Autodesk Inventor part; units mm, degrees
ref_plane "YZ Plane" through (0, 0, 0) normal (1, 0, 0) x (0, 1, 0)
ref_plane "XZ Plane" through (0, 0, 0) normal (0, 1, 0) x (-1, 0, 0)
ref_plane "XY Plane" through (0, 0, 0) normal (0, 0, 1) x (1, 0, 0)
sketch "Sketch1" plane through (0, 0, 0) normal (0, 1, 0) x (-1, 0, 0)
  point P0 (0, 0)
sketch "Sketch2" plane through (0, 0, 0) normal (0, 1, 0) x (-1, 0, 0)
  circle A0 centre (0, 0) radius 6.35 construction
  circle A1 centre (0, -44.45) radius 38.1 construction
  circle A2 centre (0, 0) radius 25.4 construction
  circle A3 centre (17.9605, -17.9605) radius 2.4892 construction
  circle A4 centre (25.4, 0) radius 2.4892 construction
  circle A5 centre (17.9605, 17.9605) radius 2.4892 construction
  circle A6 centre (0, 25.4) radius 2.4892 construction
  circle A7 centre (-17.9605, 17.9605) radius 2.4892 construction
  circle A8 centre (-25.4, 0) radius 2.4892 construction
  circle A9 centre (-17.9605, -17.9605) radius 2.4892 construction
  circle A10 centre (0, -25.4) radius 2.4892 construction
  circle A11 centre (0, -88.9) radius 25.4 construction
  circle A12 centre (0, -88.9) radius 6.35 construction
  circle A13 centre (-17.9605, -70.9395) radius 2.4892 construction
  circle A14 centre (-25.4, -88.9) radius 2.4892 construction
  circle A15 centre (-17.9605, -106.8605) radius 2.4892 construction
  circle A16 centre (0, -114.3) radius 2.4892 construction
  circle A17 centre (17.9605, -106.8605) radius 2.4892 construction
  circle A18 centre (25.4, -88.9) radius 2.4892 construction
  circle A19 centre (17.9605, -70.9395) radius 2.4892 construction
  circle A20 centre (0, -63.5) radius 2.4892 construction
  circle A21 centre (0, 0) radius 9.525 construction
  circle A22 centre (0, -88.9) radius 9.525 construction
  circle A23 centre (47.3968, -12.5178) radius 6.35 construction
  circle A24 centre (47.3968, -76.3822) radius 6.35 construction
  circle A25 centre (-47.3968, -76.3822) radius 6.35 construction
  circle A26 centre (0, 0) radius 29.972 construction
  circle A27 centre (0, -88.9) radius 29.972 construction
  circle A28 centre (-47.3968, -12.5178) radius 6.35 construction
  circle A29 centre (47.3968, -12.5178) radius 2.4892
  circle A30 centre (47.3968, -76.3822) radius 2.4892
  circle A31 centre (-47.3968, -12.5178) radius 2.4892
  circle A32 centre (-47.3968, -76.3822) radius 2.4892
  line L0 (42.1305, -72.8341) -> (31.5979, -65.7381) construction
  line L1 (41.2573, -78.0036) -> (28.9784, -81.2466) construction
  line L2 (-41.2573, -78.0036) -> (-28.9784, -81.2466) construction
  line L3 (-42.1305, -72.8341) -> (-31.5979, -65.7381) construction
  line L4 (-41.2573, -10.8964) -> (-28.9784, -7.6534) construction
  line L5 (-42.1305, -16.0659) -> (-31.5979, -23.1619) construction
  line L6 (41.2573, -10.8964) -> (28.9784, -7.6534) construction
  line L7 (42.1305, -16.0659) -> (31.5979, -23.1619) construction
  circle A33 centre (0, -44.45) radius 14.351
  line L8 (47.3968, -82.7322) -> (-47.3968, -82.7322)
  line L9 (-53.7468, -76.3822) -> (-53.7468, -12.5178)
  line L10 (-47.3968, -6.1678) -> (47.3968, -6.1678)
  line L11 (53.7468, -12.5178) -> (53.7468, -76.3822)
  arc A34 (53.7468, -12.5178) -> (47.3968, -6.1678) centre (47.3968, -12.5178) ccw
  arc A35 (-53.7468, -76.3822) -> (-47.3968, -82.7322) centre (-47.3968, -76.3822) ccw
  arc A36 (-47.3968, -6.1678) -> (-53.7468, -12.5178) centre (-47.3968, -12.5178) ccw
  arc A37 (47.3968, -82.7322) -> (53.7468, -76.3822) centre (47.3968, -76.3822) ccw
  point P0 (-20.6699, 21.7043)
  point P1 (-20.6699, -110.6043)
  point P2 (51.7761, -80.9805)
  point P3 (51.7761, -7.9195)
  point P4 (-47.3968, -82.7322)
  dimension "d2" = 50.8
  dimension "d0" = 12.7
  dimension "d1" = 76.2
  dimension "d3" = 4.9784
  dimension "d6" = 360
  dimension "d8" = 4.9784
  dimension "d11" = 360
  dimension "d13" = 19.05
  dimension "d14" = 19.05
  dimension "d15" = 59.944
  dimension "d16" = 59.944
  dimension "d17" = 12.7
  dimension "d18" = 4.9784
  dimension "d24" = 12.7
  dimension "d25" = 28.702
extrude "Extrusion2" add sketch "Sketch2" along normal blind 6.35
properties part number "Top Plate" material "Aluminum 6061"
Model file for the job. Use its own axes, mm. Coordinates: 2 decimals unless noted, no trailing zeros. Write each loop counter-clockwise with the first axis right and the second up, starting at its lowest first coordinate (ties: lowest second). Pieces come first, ordered by that corner, then holes. Notation, with made-up numbers: (77, 4.25) - (86, 4.25) arc R26 cw to (86, 37.25) - close; hole circle Ø5 at (18, 0.5). An arc over 180 degrees is marked (long way). One line per item, written item: value. Start each with the question number.
1. Slice it at C-C (z = -44.45). Write the cut outline in (x, y), plus the area to 3 significant figures.
2. Slice it at B-B (x = 0). Write the cut outline in (y, z).
3. Flat gauge pin, fed straight in: pin 1 (3 mm diameter, centred on x = -47.4, z = -76.38, fed in from -Y). Where does the tip first touch, or does it go through?
4. Probe line 1 (Z direction, x = 0, y = 5); line 2 (Z direction, x = -47, y = 5.75); line 3 (X direction, y = 1.5, z = -11.5). List the from-to ranges inside material, lowest first. Write a range as from..to.
5. Mould opens along Z. For faces 1 (the flat face through (-53.747, 3, -44)), 2 (the cylindrical face through (49.2, 3.1, -78.1)), 3 (the flat face through (-1, 3, -82.732)) say: released by +Z, released by -Z, zero draft, split by the parting line, or undercut.
6. Slice it at A-A (y = 4). Write the cut outline in (x, z).
Answers below:
1. outline: (-53.75, 0) - (-14.35, 0) - (-14.35, 6.35) - (-53.75, 6.35) - close; (14.35, 0) - (53.75, 0) - (53.75, 6.35) - (14.35, 6.35) - close
1. area: 500 mm^2
2. outline: (0, -82.73) - (6.35, -82.73) - (6.35, -58.8) - (0, -58.8) - close; (0, -30.1) - (6.35, -30.1) - (6.35, -6.17) - (0, -6.17) - close
3. pin 1: passes through
4. line 1: z = -82.73..-58.8, -30.1..-6.17
4. line 2: z = -82.73..-78.84, -73.92..-14.98, -10.06..-6.17
4. line 3: x = -53.66..-49.67, -45.13..45.13, 49.67..53.66
5. face 1: zero draft
5. face 2: undercut
5. face 3: released by -Z
6. outline: (-53.75, -76.38) arc R6.35 ccw to (-47.4, -82.73) - (47.4, -82.73) arc R6.35 ccw to (53.75, -76.38) - (53.75, -12.52) arc R6.35 ccw to (47.4, -6.17) - (-47.4, -6.17) arc R6.35 ccw to (-53.75, -12.52) - close; hole circle Ø4.98 at (-47.4, -76.38); hole circle Ø4.98 at (-47.4, -12.52); hole circle Ø28.7 at (0, -44.45); hole circle Ø4.98 at (47.4, -76.38); hole circle Ø4.98 at (47.4, -12.52)
